from build123d import *

# Parameters (mm, degrees)
ESQUISSE10_W            = 10.105828541
ESQUISSE10_H            = 38
BOSS_EXTRU_1_DEPTH      = 2.5
ESQUISSE13_R            = 1.8
ENL_V_MAT_EXTRU_1_DEPTH = 2.5
BOSS_EXTRU_2_REACH      = 51.459
ESQUISSE16_W            = 9
ESQUISSE16_H            = 38
NERVURE3_REACH          = 51.459
ESQUISSE17_WALL_W       = 106.880712272
ESQUISSE17_WALL_H       = 38


with BuildPart() as part:
    # Esquisse12 → Lissage4 section 0
    with BuildSketch(Plane(origin=(0, 0, 0), x_dir=(-1, 0, 0), z_dir=(0, 0, -1))):
        with BuildLine():
            Line((0, -19), (0, 19))
            Line((0, 19), (6.966679003, 45))
            Line((6.966679003, 45), (10.072507544, 45))
            Line((10.072507544, 45), (3.105828541, 19))
            Line((3.105828541, 19), (3.105828541, -19))
            Line((3.105828541, -19), (10.072507544, -45))
            Line((10.072507544, -45), (6.966679003, -45))
            Line((6.966679003, -45), (0, -19))
        make_face()
    # Esquisse11 → Lissage4 section 1
    with BuildSketch(Plane.XY.offset(-14.75)):
        with BuildLine():
            Line((-11.162831426, 45), (-14.268659967, 45))
            Line((-14.268659967, 45), (-8.105828541, 22))
            Line((-8.105828541, 22), (-8.105828541, -22))
            Line((-8.105828541, -22), (-14.268659967, -45))
            Line((-14.268659967, -45), (-11.162831426, -45))
            Line((-11.162831426, -45), (-5, -22))
            Line((-5, -22), (-5, 22))
            Line((-5, 22), (-11.162831426, 45))
        make_face()
    loft()



with BuildPart() as body_2:
    # Esquisse10 → Boss.-Extru.1 (new body)
    with BuildSketch(Plane.XY):
        with Locations((1.947085729, 0)):
            Rectangle(ESQUISSE10_W, ESQUISSE10_H)
    extrude(amount=-BOSS_EXTRU_1_DEPTH)

    # Esquisse13 → Enlèv. mat.-Extru.1 (cut)
    with BuildSketch(Plane.XY):
        with Locations((3.5, 15.5)):
            Circle(ESQUISSE13_R)
        with Locations((3.5, -15.5)):
            Circle(ESQUISSE13_R)
    extrude(amount=-ENL_V_MAT_EXTRU_1_DEPTH, mode=Mode.SUBTRACT)


with BuildPart() as part_1:
    add(part.part)

    add(body_2.part)  # Boss.-Extru.2 merges body 2
    # Boss.-Extru.2: up to this plane
    boss_extru_2_end = Plane(origin=(0, 0, 0), z_dir=(0.9470658794157988, 0, -0.32103928115789765))
    # Esquisse16 → Boss.-Extru.2 (add, up to the surface)
    with BuildSketch(Plane(origin=(0, 0, 0), x_dir=(0, 0, -1), z_dir=(1, 0, 0)), mode=Mode.PRIVATE) as boss_extru_2_sk1:
        with Locations((7, 0)):
            Rectangle(ESQUISSE16_W, ESQUISSE16_H)
    boss_extru_2_tool1 = split(extrude(boss_extru_2_sk1.sketch, amount=-BOSS_EXTRU_2_REACH, mode=Mode.PRIVATE), bisect_by=boss_extru_2_end, keep=Keep.BOTH, mode=Mode.PRIVATE)
    add(boss_extru_2_tool1.solids().sort_by_distance((0, 0, -7))[0])

    # Esquisse17 wall → Nervure3 (add, up to next)
    with BuildSketch(Plane(origin=(-2.5, 0, -13.125), x_dir=(-0.838443616301, 0, -0.544988350595), z_dir=(-0.544988350595, 0, 0.838443616301)), mode=Mode.PRIVATE) as nervure3_sk1:
        Rectangle(ESQUISSE17_WALL_W, ESQUISSE17_WALL_H)
    nervure3_tool1 = extrude(nervure3_sk1.sketch, amount=NERVURE3_REACH, mode=Mode.PRIVATE) - part_1.part
    add(nervure3_tool1.solids().sort_by_distance((-2.5, 0, -13.125))[0])


solid = part_1.part
The listing builds one solid part. Answer for the finished solid, in the listing's coordinates (mm). A direction names the side the tool comes from. Give positions to 0.01 mm unless a question says otherwise; leave off trailing zeros. Write each loop counter-clockwise with the first axis right and the second up, starting at its lowest first coordinate (ties: lowest second). Pieces come first, ordered by that corner, then holes. Notation, with made-up numbers: (77, 25.25) -> (127, 25.25) arc R8 cw to (127, 39.25) -> close; hole circle Ø7 at (-21, 18). An arc over 180 degrees is marked (long way). One line per question, with ' | ' between items. Start each with the question number.
1. Section A-A (x = 3.5) is taken. Determine the outline of the cut face in (y, z), plus the area to 3 significant figures.
2. For faces 1 (the flat face through (-0.4, 19, -6.4)), 2 (the flat face through (3, 0, -2.5)), 3 (the flat face through (7, 0, -1)), determine the directions among +Z, -Z, +X, -X, +Y, -Y from which every point of the face is accessible in a straight line to the end or side of a thin tool.
3. Given pin 1 Ø4.5 at (y, z) = (1, -7) entering from +X; pin 2 Ø6 at (y, z) = (21.5, -5) entering from -X; pin 3 Ø10 at (x, y) = (1, 1) entering from +Z; pin 4 Ø5.5 at (x, y) = (2, 2.5) entering from -Z, each flat-ended and moving along its own axis, determine where each tip first touches the part or whether it passes through.
4. Find the intervals of material crossed by probe 1 along Y at (x, z) = (3.5, -1.35); probe 2 along Z at (x, y) = (6, -7.5); probe 3 along X at (y, z) = (10, -0.75), in increasing order.
5. For a pull along Y with two mould halves and no side action, classify faces 4 (the flat face through (0, 0, -7)), 5 (the cylindrical face through (4.468, 17.018, -1.232)), 6 (the flat face through (-0.4, -19, -6.4)), 7 (the cylindrical face through (4.468, -13.982, -1.232)) as pulls with the +Y half, pulls with the -Y half, needs draft (parallel to the pull), parting line crosses it, or undercut.
6. Section B-B (z = -1.5) is taken. State how many separate pieces and enclosed holes the cut face has, plus the area to 3 significant figures.
Response values:
1) outline: (-19, -2.5) -> (-17.3, -2.5) -> (-17.3, 0) -> (-19, 0) -> close; (-13.7, -2.5) -> (13.7, -2.5) -> (13.7, 0) -> (-13.7, 0) -> close; (17.3, -2.5) -> (19, -2.5) -> (19, 0) -> (17.3, 0) -> close | area: 77.0 mm2
2) face 1: -Z, +X, +Y | face 2: -Z, +X, +Y, -Y | face 3: +Z, -Z, +X, +Y, -Y
3) pin 1: x = 0 | pin 2: x = -6.37 | pin 3: z = 0 | pin 4: z = -11.99
4) probe 1: -19 to -17.3, -13.7 to 13.7, 17.3 to 19 | probe 2: -2.5 to 0 | probe 3: -3.36 to 7
5) face 4: needs draft | face 5: undercut | face 6: pulls with the -Y half | face 7: undercut
6) separate pieces: 1 | enclosed holes: 2 | area: 544 mm2
